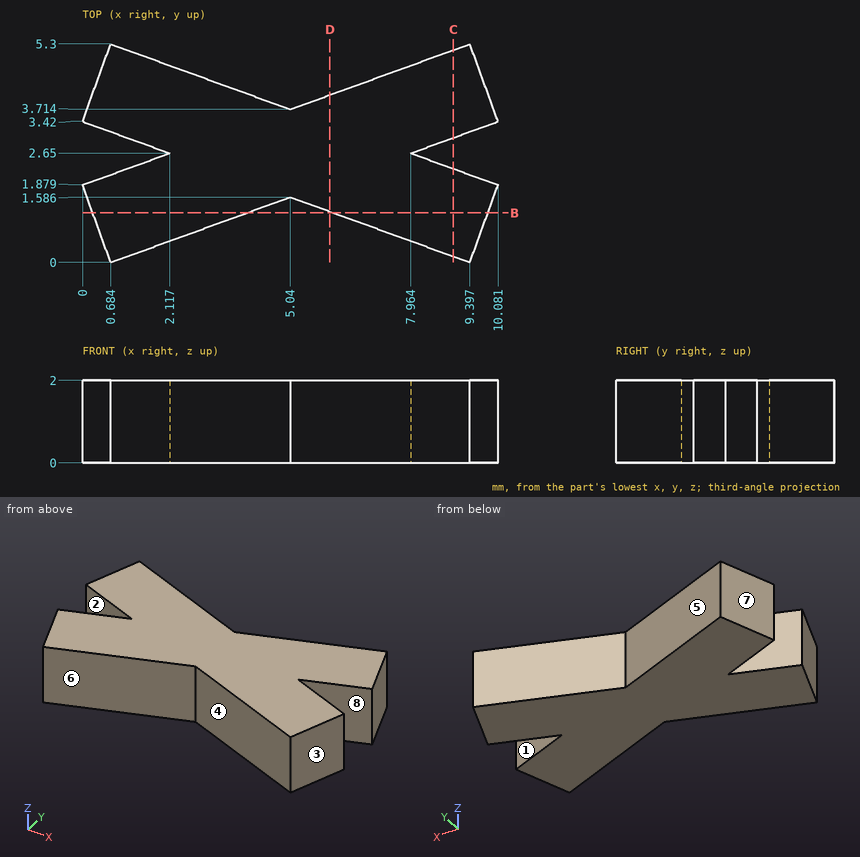
Can you work these out from the drawing? Everything is in mm from the part's minimum corner. A direction names the side the tool comes from. Coordinates: 2 decimals unless noted, no trailing zeros. Loops run counter-clockwise (first coordinate to the right, second up) from the corner with the lowest first, then second, coordinate; pieces in that order, holes last.
1) Which directions (+Z, -Z, +X, -X, +Y, -Y) give clear straight access to the entire face, cutting with the end or side of a thin tool? Please do the marked faces 1, 2, 3, 4 and 5.
2) Imagine slicing it at D-D on x = 6. List the corners of the cut face in (y, z) for me.
3) Imagine slicing it at C-C on x = 9. List the corners of the cut face in (y, z) for me (1 decimal).
4) Imagine slicing it at B-B on y = 1.2. List the corners of the cut face in (x, z) for me.
5) I need wall thicknesses on probe 1 along Y at (x, z) = (9.25, 1.5) (1 decimal); probe 2 along Y at (x, z) = (8.5, 1.4) (1 decimal); probe 3 along Y at (x, z) = (3.5, 1.4) (1 decimal). Which ranges of each line are inside material? Lowest first, please.
6) Thinking about a two-plate mould opening in X: for the marked faces 6, 7 and 8, which applies, pulls with the +X half, pulls with the -X half, needs draft (parallel to the pull), parting line crosses it, or undercut?
Completed:
1. face 1: +Z, -Z, +X
1. face 2: +Z, -Z, -X
1. face 3: +Z, -Z, +X, -Y
1. face 4: +Z, -Z, -Y
1. face 5: +Z, -Z, +Y
2. outline: (1.24, 0) - (4.06, 0) - (4.06, 2) - (1.24, 2) - close
3. outline: (0.1, 0) - (2.3, 0) - (2.3, 2) - (0.1, 2) - close; (3, 0) - (5.2, 0) - (5.2, 2) - (3, 2) - close
4. outline: (0.25, 0) - (3.98, 0) - (3.98, 2) - (0.25, 2) - close; (6.1, 0) - (9.83, 0) - (9.83, 2) - (6.1, 2) - close
5. probe 1: y = 0.1 to 2.2, 3.1 to 5.2
5. probe 2: y = 0.3 to 2.5, 2.8 to 5
5. probe 3: y = 1 to 4.3
6. face 6: undercut
6. face 7: pulls with the -X half
6. face 8: pulls with the +X half
